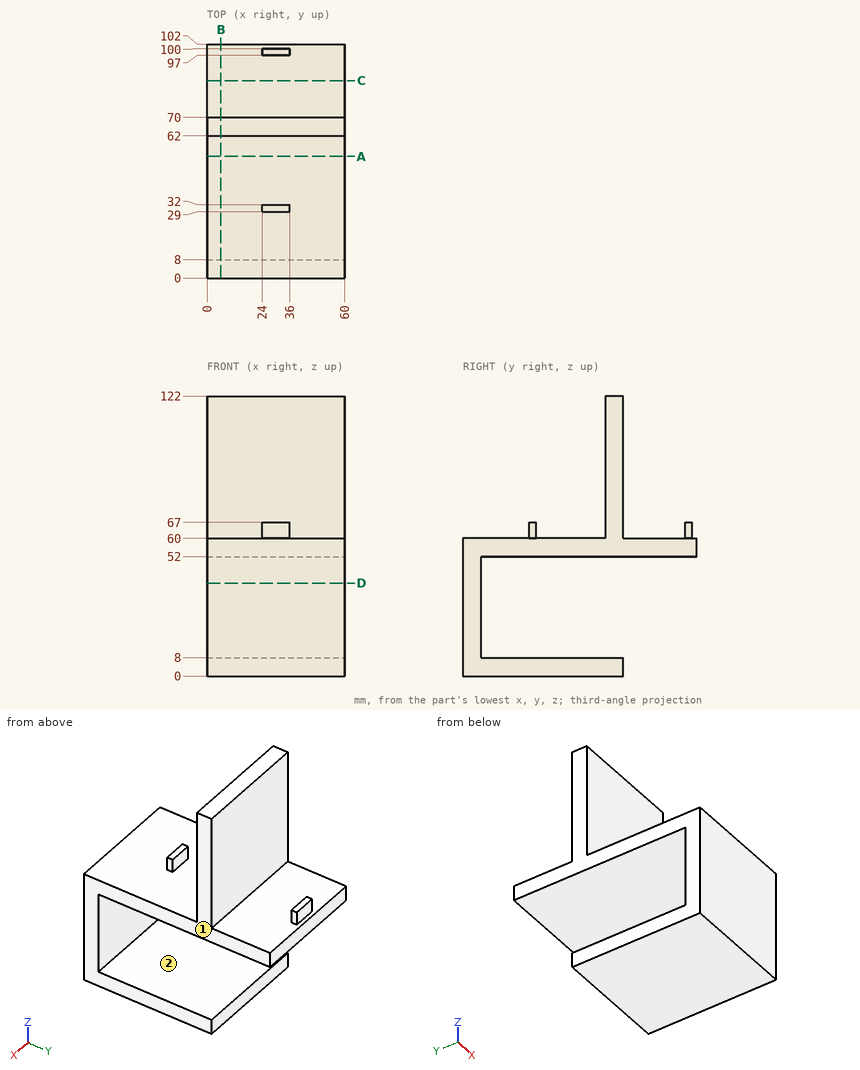
Here's the drawing with two shaded views (mm, measured from the low corner). I have some questions. A direction names the side the tool comes from. Round coordinates to 2 decimals unless told otherwise and drop trailing zeros. Loops run counter-clockwise (first coordinate to the right, second up) from the corner with the lowest first, then second, coordinate; pieces in that order, holes last.
Item 1: Which directions (+Z, -Z, +X, -X, +Y, -Y) give clear straight access to the entire face, cutting with the end or side of a thin tool? Please do the marked faces 1 and 2.
Item 2: Suppose I cut it at A-A, the plane y = 53. Write out the boundary of the cut face in (x, z), then the cut area to 3 significant figures.
Item 3: Will these pins go through, and if not, where does the flat tip stop? pin 1 Ø9 at (x, z) = (27.5, 2.5) entering from +Y; pin 2 Ø1.5 at (y, z) = (98, 63) entering from +X; pin 3 Ø2 at (x, z) = (29.5, 64.5) entering from -Y.
Item 4: Please list where these lines run through material, in increasing order: L1, parallel to Z at x = 27.5, y = 20.5; L2, parallel to Z at x = 32.5, y = 66; L3, parallel to Y at x = 14, z = 63.5.
Item 5: Suppose I cut it at D-D, the plane z = 40.5. Write out the boundary of the cut face in (x, y).
Item 6: Suppose I cut it at B-B, the plane x = 6. Write out the boundary of the cut face in (y, z), then the cut area to 3 significant figures.
Item 7: Suppose I cut it at C-C, the plane y = 86. Write out the boundary of the cut face in (x, z), then the cut area to 3 significant figures.
Reported:
1. face 1: +Z, -Z, +X, +Y, -Y
1. face 2: +X, -X, +Y
2. outline: (0, 0) - (60, 0) - (60, 8) - (0, 8) - close; (0, 52) - (60, 52) - (60, 60) - (0, 60) - close
2. area: 960 mm2
3. pin 1: stops at y = 70
3. pin 2: stops at x = 36
3. pin 3: stops at y = 29
4. L1: z = 0 to 8, 52 to 60
4. L2: z = 0 to 8, 52 to 122
4. L3: y = 62 to 70
5. outline: (0, 0) - (60, 0) - (60, 8) - (0, 8) - close
6. outline: (0, 0) - (70, 0) - (70, 8) - (8, 8) - (8, 52) - (102, 52) - (102, 60) - (70, 60) - (70, 122) - (62, 122) - (62, 60) - (0, 60) - close
6. area: 2,220 mm2
7. outline: (0, 52) - (60, 52) - (60, 60) - (0, 60) - close
7. area: 480 mm2
